from build123d import *

# Parameters (mm, degrees)
F1_DEPTH     = 20
F2_DEPTH     = 5
F3_R         = 4.75
F4_DEPTH     = 10
F5_R         = 1.4
F6_DEPTH     = 5.4620024133
F7_T1_DEPTH  = 37.5
F7_T3_DEPTH  = 22.5
F7_T5_DEPTH  = 69.5
F7_T7_DEPTH  = 84.5
F7_T9_DEPTH  = 10
F7_S13_W     = 5
F7_S13_H     = 5
F7_T14_DEPTH = 5
F7_S19_W     = 5
F7_S19_H     = 5
F7_T20_DEPTH = 5
F7_T27_DEPTH = 35
F7_T31_DEPTH = 82
F7_T38_DEPTH = 35
F7_T42_DEPTH = 82


# Not quite as in the source:
# - a fillet or chamfer that OpenCascade refuses, or shapes differently, is made with other operations: its cross-section is extruded or revolved along the edge and cut away or added


with BuildPart() as f1:
    # F0 (on Top) → F1 (new body)
    with BuildSketch(Plane.XY):
        Polygon((0, 10), (0, 0), (0, -10), (10, -10), (10, -67), (30, -67), (30, 10), align=None)
        Polygon((25.5, -61), (25.5, -66.5), (20, -66.5), (14.5, -66.5), (14.5, -61), align=None, mode=Mode.SUBTRACT)
    extrude(amount=F1_DEPTH)

    # F0 (on Top) → F2 (join)
    with BuildSketch(Plane.XY):
        Polygon((20, -66.5), (25.5, -66.5), (25.5, -61), (14.5, -61), (14.5, -66.5), align=None)
    extrude(amount=F2_DEPTH)

    # F3 (on face) → F4 (cut)
    with BuildSketch(Plane(origin=(0, 0, 0), x_dir=(0, -1, 0), z_dir=(-1, 0, 0))):
        with Locations((0, 10)):
            Circle(F3_R)
    extrude(amount=-F4_DEPTH, mode=Mode.SUBTRACT)

    # F5 (on face) → F6 (cut, through all)
    with BuildSketch(Plane(origin=(0, 10, 0), x_dir=(-1, 0, 0), z_dir=(0, 1, 0))):
        with Locations((-5, 10)):
            Circle(F5_R)
    extrude(amount=-F6_DEPTH, mode=Mode.SUBTRACT)

    # F7: fillet of radius 5 on 9 edges, made by hand

    # F7_s2 → F7_t1 (cut)
    with BuildSketch(Plane.YZ.offset(-12.5)):
        with BuildLine():
            ThreePointArc((10, 15), (8.5355339059, 18.5355339059), (5, 20))
            Line((5, 20), (10, 20))
            Line((10, 20), (10, 15))
        make_face()
        with BuildLine():
            ThreePointArc((10, 5), (8.5355339059, 1.4644660941), (5, 0))
            Line((5, 0), (10, 0))
            Line((10, 0), (10, 5))
        make_face()
    extrude(amount=F7_T1_DEPTH, mode=Mode.SUBTRACT)

    # F7_s4 → F7_t3 (cut)
    with BuildSketch(Plane.YZ.offset(-12.5)):
        with BuildLine():
            ThreePointArc((-5, 20), (-8.5355339059, 18.5355339059), (-10, 15))
            Line((-10, 15), (-10, 20))
            Line((-10, 20), (-5, 20))
        make_face()
        with BuildLine():
            ThreePointArc((-5, 0), (-8.5355339059, 1.4644660941), (-10, 5))
            Line((-10, 5), (-10, 0))
            Line((-10, 0), (-5, 0))
        make_face()
    extrude(amount=F7_T3_DEPTH, mode=Mode.SUBTRACT)

    # F7_s6 → F7_t5 (cut)
    with BuildSketch(Plane.XZ.offset(10)):
        with BuildLine():
            ThreePointArc((15, 20), (11.4644660941, 18.5355339059), (10, 15))
            Line((10, 15), (10, 20))
            Line((10, 20), (15, 20))
        make_face()
        with BuildLine():
            ThreePointArc((15, 0), (11.4644660941, 1.4644660941), (10, 5))
            Line((10, 5), (10, 0))
            Line((10, 0), (15, 0))
        make_face()
    extrude(amount=F7_T5_DEPTH, mode=Mode.SUBTRACT)

    # F7_s8 → F7_t7 (cut)
    with BuildSketch(Plane.XZ.offset(-5)):
        with BuildLine():
            ThreePointArc((25, 20), (28.5355339059, 18.5355339059), (30, 15))
            Line((30, 15), (30, 20))
            Line((30, 20), (25, 20))
        make_face()
        with BuildLine():
            ThreePointArc((25, 0), (28.5355339059, 1.4644660941), (30, 5))
            Line((30, 5), (30, 0))
            Line((30, 0), (25, 0))
        make_face()
    extrude(amount=F7_T7_DEPTH, mode=Mode.SUBTRACT)

    # F7_s10 → F7_t9 (cut)
    with BuildSketch(Plane.XY.offset(5)):
        with BuildLine():
            ThreePointArc((25, 10), (28.5355339059, 8.5355339059), (30, 5))
            Line((30, 5), (30, 10))
            Line((30, 10), (25, 10))
        make_face()
    extrude(amount=F7_T9_DEPTH, mode=Mode.SUBTRACT)


with BuildPart() as f7_tool12:
    # F7_s13 → F7_t14 (new body)
    with BuildSketch(Plane.XZ.offset(-5)):
        with Locations((27.5, 17.5)):
            Rectangle(F7_S13_W, F7_S13_H)
    extrude(amount=-F7_T14_DEPTH)

    # F7_s15 → F7_t16 (revolve, cut)
    with BuildSketch(Plane(origin=(25, 5, 15), x_dir=(-0.7071067812, 0, -0.7071067812), z_dir=(0.7071067812, 0, -0.7071067812))):
        with BuildLine():
            ThreePointArc((0, -5), (5, 0), (0, 5))
            Line((0, 5), (0, -5))
        make_face()
    revolve(axis=Axis((25, 5, 15), (0, 1, 0)), mode=Mode.SUBTRACT)


with BuildPart() as f1_1:
    add(f1.part)

    # F7_t11: cut F7_tool12
    add(f7_tool12.part, mode=Mode.SUBTRACT)


with BuildPart() as f7_tool18:
    # F7_s19 → F7_t20 (new body)
    with BuildSketch(Plane.XZ.offset(-5)):
        with Locations((27.5, 2.5)):
            Rectangle(F7_S19_W, F7_S19_H)
    extrude(amount=-F7_T20_DEPTH)

    # F7_s21 → F7_t22 (revolve, cut)
    with BuildSketch(Plane(origin=(25, 5, 5), x_dir=(-0.7071067812, 0, 0.7071067812), z_dir=(-0.7071067812, 0, -0.7071067812))):
        with BuildLine():
            ThreePointArc((0, -5), (5, 0), (0, 5))
            Line((0, 5), (0, -5))
        make_face()
    revolve(axis=Axis((25, 5, 5), (0, 1, 0)), mode=Mode.SUBTRACT)


with BuildPart() as f1_2:
    add(f1_1.part)

    # F7_t17: cut F7_tool18
    add(f7_tool18.part, mode=Mode.SUBTRACT)


with BuildPart() as f7_tool25:
    # F7_s26 → F7_t27 (new body)
    with BuildSketch(Plane.YZ.offset(-12.5)):
        with BuildLine():
            ThreePointArc((-5, 20), (-8.5355339059, 18.5355339059), (-10, 15))
            Line((-10, 15), (-10, 20))
            Line((-10, 20), (-5, 20))
        make_face()
    extrude(amount=F7_T27_DEPTH)

    split(bisect_by=Plane.YZ.offset(10), keep=Keep.TOP)


with BuildPart() as f7_tool29:
    # F7_s30 → F7_t31 (new body)
    with BuildSketch(Plane.XZ.offset(-2.5)):
        with BuildLine():
            ThreePointArc((15, 20), (11.4644660941, 18.5355339059), (10, 15))
            Line((10, 15), (10, 20))
            Line((10, 20), (15, 20))
        make_face()
    extrude(amount=F7_T31_DEPTH)

    split(bisect_by=Plane.XZ.offset(10), keep=Keep.BOTTOM)


with BuildPart() as f7_tool25_1:
    add(f7_tool25.part)

    # F7_t33: intersect F7_tool29
    add(f7_tool29.part, mode=Mode.INTERSECT)


with BuildPart() as f1_3:
    add(f1_2.part)

    # F7_t23: cut F7_tool25
    add(f7_tool25_1.part, mode=Mode.SUBTRACT)


with BuildPart() as f7_tool36:
    # F7_s37 → F7_t38 (new body)
    with BuildSketch(Plane.YZ.offset(-12.5)):
        with BuildLine():
            ThreePointArc((-5, 0), (-8.5355339059, 1.4644660941), (-10, 5))
            Line((-10, 5), (-10, 0))
            Line((-10, 0), (-5, 0))
        make_face()
    extrude(amount=F7_T38_DEPTH)

    split(bisect_by=Plane.YZ.offset(10), keep=Keep.TOP)


with BuildPart() as f7_tool40:
    # F7_s41 → F7_t42 (new body)
    with BuildSketch(Plane.XZ.offset(-2.5)):
        with BuildLine():
            ThreePointArc((15, 0), (11.4644660941, 1.4644660941), (10, 5))
            Line((10, 5), (10, 0))
            Line((10, 0), (15, 0))
        make_face()
    extrude(amount=F7_T42_DEPTH)

    split(bisect_by=Plane.XZ.offset(10), keep=Keep.BOTTOM)


with BuildPart() as f7_tool36_1:
    add(f7_tool36.part)

    # F7_t44: intersect F7_tool40
    add(f7_tool40.part, mode=Mode.INTERSECT)


with BuildPart() as f1_4:
    add(f1_3.part)

    # F7_t34: cut F7_tool36
    add(f7_tool36_1.part, mode=Mode.SUBTRACT)


solid = f1_4.part
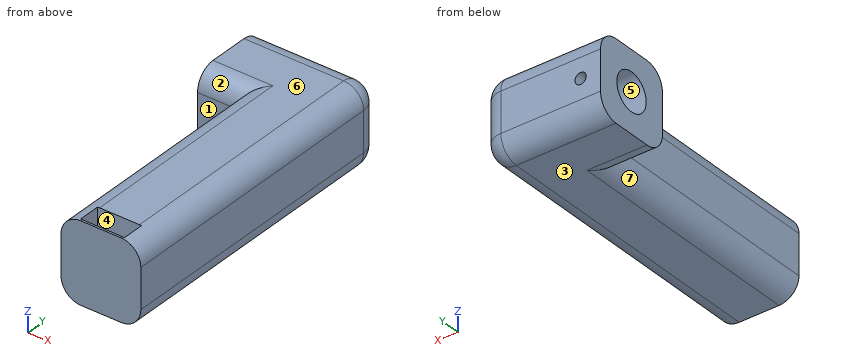
Source: CAD feature listing. Evaluate the final solid. Frame: model axes, mm. Face numbers are marked on the shaded views. A direction names the side the tool comes from. Coordinates: 2 decimals unless noted, no trailing zeros. Order: outer loops, then holes, each group sorted by start corner. A loop starts at its lowest first (then second) coordinate and runs counter-clockwise, first axis right, second up. Notation, with made-up numbers: M -28.5,12 L -21.5,12 A22 cw -21.5,18 Z; hole C 50,69.25 d11. An arc over 180 degrees is marked long. Write each question's results on one line, items separated by ' | '. Start each with the question number.
1. Material intervals for L1, parallel to Y at x = 19, z = 8.25; L2, parallel to X at y = 4, z = 8; L3, parallel to Z at x = 5, y = 6.25, sorted ascending.
2. Section C-C, the plane x = 5. Return the cut outline in (y, z), then the cut area to 3 significant figures.
3. Reachability of the marked faces 1, 2 and 3 from +Z, -Z, +X, -X, +Y, -Y: full face, straight path, thin tool, end or side. Return the list, or none.
4. Draft query along Z for the marked faces 4, 5, 6 and 7. Return one class per face: +Z half, -Z half, draft (parallel to the pull), parting line (faces both ways), or undercut.
5. Section B-B, the plane y = -54. Return the cut outline in (x, z).
6. Section D-D, the plane z = 14. Return the cut outline in (x, y).
7. Pin query (flat end, axial travel): pin 1 (2.5 mm diameter, centred on x = 5, z = 10, fed in from +Y); pin 2 (1.6 mm diameter, centred on y = -62.5, z = 14, fed in from -X). Return the tip coordinate at first contact, or that it passes through.
8. Section A-A, the plane z = 10. Return the cut outline in (x, y).
Solution:
1) L1: -67 to -66.5, -61 to 10 | L2: 10 to 30 | L3: 0.16 to 8.6, 11.4 to 19.84
2) outline: M -10,5 A5 ccw -5,0 L 5,0 A5 ccw 10,5 L 10,8.6 L 4.54,8.6 A4.75 cw long 4.54,11.4 L 10,11.4 L 10,15 A5 ccw 5,20 L -5,20 A5 ccw -10,15 Z | area: 293 mm²
3) face 1: +Z, -Z, -X, -Y | face 2: +Z, -X, -Y | face 3: -Z, +X, -X, +Y, -Y
4) face 4: draft | face 5: undercut | face 6: +Z half | face 7: -Z half
5) outline: M 10,5 A5 ccw 15,0 L 25,0 A5 ccw 30,5 L 30,15 A5 ccw 25,20 L 15,20 A5 ccw 10,15 Z
6) outline: M 0,-10 L 10,-10 L 10,-67 L 30,-67 L 30,5 A5 ccw 25,10 L 0,10 L 0,2.56 L 10,2.56 L 10,-2.56 L 0,-2.56 Z; hole M 14.5,-66.5 L 25.5,-66.5 L 25.5,-61 L 14.5,-61 Z
7) pin 1: y = -4.58 | pin 2: x = 10
8) outline: M 0,-10 L 10,-10 L 10,-67 L 30,-67 L 30,5 A5 ccw 25,10 L 6.4,10 L 6.4,4.75 L 10,4.75 L 10,-4.75 L 0,-4.75 Z; M 0,4.75 L 3.6,4.75 L 3.6,10 L 0,10 Z; hole M 14.5,-66.5 L 25.5,-66.5 L 25.5,-61 L 14.5,-61 Z
